Could you check a few things on this model? Use its own coordinates, in mm. A direction names the side the tool comes from. Give positions to 0.01 mm unless a question says otherwise; leave off trailing zeros. Loops run counter-clockwise (first coordinate to the right, second up) from the corner with the lowest first, then second, coordinate; pieces in that order, holes last. Notation, with made-up numbers: M 59,7 L 85,7 A34 ccw 85,40 Z; hole C -13.5,10 d11. An arc over 180 degrees is marked long. Return JSON: item names as keys, results as strings. Group by question number.
1. For faces 5 (the flat face through (40, -11, -25)), 6 (the cylindrical face through (89.991, 37.046, 4.769)), which set-ups out of +Z, -Z, +X, -X, +Y, -Y let a thin tool reach every point of the face, with its end or its side?
2. If we section it at B-B (x = 0): Write out the boundary of the cut face in (y, z), plus the area to 3 significant figures.
3. For pin 1 (8 mm diameter, centred on y = 13, z = -7, fed in from -X); pin 2 (4 mm diameter, centred on x = -4, z = 12.5, fed in from +Y); pin 3 (1 mm diameter, centred on y = -40, z = 8.5, fed in from +X); pin 4 (6 mm diameter, centred on x = 0, y = 0, fed in from -Z), each with a flat end and sliding along its axis, tell me the tip position at first contact or that it passes through.
4. If we mould it in two halves opening along Y, with no side actions, what happens to faces 1 (the cylindrical face through (-1.08, -4.88, 21.3)), 2 (the flat face through (45.147, -49.746, 0.35)), 3 (the cylindrical face through (-1.08, -4.88, -21.2)), 4 (the flat face through (98.85, 16, 0))? For each: +Y half, -Y half, draft (parallel to the pull), parting line (faces both ways), or undercut.
5. If we section it at C-C (z = 2): Write out the boundary of the cut face in (x, y), plus the area to 3 significant figures.
6. Please list where these lines run through material, in increasing order: line 1 (Z direction, x = 50.5, y = 30.5); line 2 (Y direction, x = 0, z = -23.5); line 3 (Y direction, x = 33, z = 6).
7. If we section it at A-A (y = 0): Write out the boundary of the cut face in (x, z), plus the area to 3 significant figures.
8. If we section it at D-D (z = -9): Write out the boundary of the cut face in (x, y), plus the area to 3 significant figures.
```python
from build123d import *

# Parameters (mm, degrees)
BOSS_EXTRU_2_DEPTH      = 25
ENL_V_MAT_EXTRU_1_DEPTH = 17.5
ESQUISSE3_R             = 5
ENL_V_MAT_EXTRU_2_DEPTH = 51
CONG_1_R                = 10
CONG_2_R                = 10
CONG_3_R                = 10
ESQUISSE5_R             = 5
ENL_V_MAT_EXTRU_3_DEPTH = 19.220103764


with BuildPart() as part:
    # Esquisse1 → Boss.-Extru.2 (new body, symmetric)
    with BuildSketch(Plane.XY):
        Polygon((-18.162962303, -86.173753074), (98.849698137, -18.845918586), (98.849698137, 60.802751576), (-13.043991627, 8.826246926), align=None)
    extrude(amount=BOSS_EXTRU_2_DEPTH, both=True)

    # Esquisse2 → Enl_v. mat.-Extru.1 (cut, symmetric)
    with BuildSketch(Plane.XY):
        Polygon((-16.815864757, -61.173753074), (82.946312501, -14.832540436), (80.711120454, 52.377076551), (-13.043991627, 8.826246926), align=None)
    extrude(amount=ENL_V_MAT_EXTRU_1_DEPTH, both=True, mode=Mode.SUBTRACT)

    # Esquisse3 → Enl_v. mat.-Extru.2 (cut, through all)
    with BuildSketch(Plane.XY.offset(25)):
        Circle(ESQUISSE3_R)
    extrude(amount=-ENL_V_MAT_EXTRU_2_DEPTH, mode=Mode.SUBTRACT)

    # Cong_1
    cong_1_edges = [part.edges().sort_by_distance(p)[0] for p in [
        (-13.043991627, 8.826246926, -21.25),
        (-13.043991627, 8.826246926, 21.25),
    ]]
    fillet(cong_1_edges, radius=CONG_1_R)

    # Cong_2
    cong_2_edges = [part.edges().sort_by_distance(p)[0] for p in [
        (-18.162962303, -86.173753074, 0),
    ]]
    fillet(cong_2_edges, radius=CONG_2_R)

    # Cong_3
    cong_3_edges = [part.edges().sort_by_distance(p)[0] for p in [
        (98.849698137, 60.802751576, 0),
        (98.849698137, -18.845918586, 0),
    ]]
    fillet(cong_3_edges, radius=CONG_3_R)

    # Esquisse5 → Enl_v. mat.-Extru.3 (cut, through all)
    with BuildSketch(Plane(origin=(82.361931549, 2.739112982, 0), x_dir=(0, 0, 1), z_dir=(-0.999447443, -0.033238651, 0))):
        with Locations((0, 32.532014282)):
            Circle(ESQUISSE5_R)
    extrude(amount=-ENL_V_MAT_EXTRU_3_DEPTH, mode=Mode.SUBTRACT)


solid = part.part
```
Answer:
{
 "1": {"face 5": "-Z, +X, -X, +Y, -Y", "face 6": "none"},
 "2": {"outline": "M -75.72,-25 L -5,-25 L -5,-17.5 L -53.36,-17.5 L -53.36,17.5 L -5,17.5 L -5,25 L -75.72,25 Z; M 5,-25 L 14.89,-25 L 14.89,-17.5 L 5,-17.5 Z; M 5,17.5 L 14.89,17.5 L 14.89,25 L 5,25 Z", "area": "1,990 mm²"},
 "3": {"pin 1": "stops at x = 81.89", "pin 2": "stops at y = -54.29", "pin 3": "stops at x = 62.95", "pin 4": "passes through"},
 "4": {"face 1": "undercut", "face 2": "-Y half", "face 3": "undercut", "face 4": "draft"},
 "5": {"outline": "M -17.17,-67.78 A10 ccw -2.2,-76.99 L 93.84,-21.73 A10 ccw 98.85,-13.06 L 98.85,31.25 L 81.43,30.67 L 82.95,-14.83 L -16.82,-61.17 Z; M 80.71,52.38 L 81.13,39.83 L 98.85,40.42 L 98.85,45.13 A10 ccw 84.64,54.2 Z", "area": "2,940 mm²"},
 "6": {"line 1": "z = -25 to -17.5, 17.5 to 25", "line 2": "y = -75.72 to -5, 5 to 14.89", "line 3": "y = -56.74 to -38.03"},
 "7": {"outline": "M -13.52,-25 L -5,-25 L -5,-17.5 L -13.52,-17.5 Z; M -13.52,17.5 L -5,17.5 L -5,25 L -13.52,25 Z; M 5,-25 L 98.85,-25 L 98.85,25 L 5,25 L 5,17.5 L 82.45,17.5 L 82.45,-17.5 L 5,-17.5 Z", "area": "2,110 mm²"},
 "8": {"outline": "M -17.17,-67.78 A10 ccw -2.2,-76.99 L 93.84,-21.73 A10 ccw 98.85,-13.06 L 98.85,45.13 A10 ccw 84.64,54.2 L 80.71,52.38 L 82.95,-14.83 L -16.82,-61.17 Z", "area": "3,100 mm²"}
}
